Could you check a few things on this model? Use its own coordinates, in mm. A direction names the side the tool comes from. Round coordinates to 2 decimals unless told otherwise and drop trailing zeros. Write each loop counter-clockwise with the first axis right and the second up, starting at its lowest first coordinate (ties: lowest second). Pieces come first, ordered by that corner, then holes. Notation, with made-up numbers: (84, 58) - (123, 58) arc R19 ccw to (123, 79) - close; hole circle Ø4 at (39.25, 5.25). An arc over 180 degrees is marked (long way). Put each result on its own line as item: value.
from build123d import *

# Parameters (mm, degrees)
BOX023_W                 = 4
BOX023_H                 = 9
BOX023_DEPTH             = 3
PRISM015_DEPTH           = 10
PRISM015_ROLL_ANGLE      = -90.000052
PRISM015_PITCH_ANGLE     = -59.999967
PRISM015_PLACEMENT_ANGLE = 90.000052
CYLINDER032_R            = 1.75
CYLINDER032_DEPTH        = 68
CYLINDER032_PITCH_ANGLE  = 90
BOX022_W                 = 6
BOX022_H                 = 9
BOX022_DEPTH             = 11
CHAMFER020_SIZE          = 1.5
FILLET015_R              = 1.5
BOX021_W                 = 12
BOX021_H                 = 16
BOX021_DEPTH             = 10
CYLINDER033_R            = 2
CYLINDER033_DEPTH        = 15
PAD035009_DEPTH          = 35
CYLINDER034_R            = 1.75
CYLINDER034_DEPTH        = 50
PRISM012_DEPTH           = 10
SKETCH031_W              = 88
SKETCH031_H              = 83
PAD035007_DEPTH          = 2
SKETCH032_W              = 58
SKETCH032_H              = 72
PAD035008_DEPTH          = 6
BOX020_W                 = 92
BOX020_H                 = 87
BOX020_DEPTH             = 6
CHAMFER019_SIZE          = 1


with BuildPart() as cubo022:
    # Box023 → Box023 (new body)
    with BuildSketch(Plane(origin=(-29.75, -4.5, 23), x_dir=(1, 0, 0), z_dir=(0, 0, 1))):
        with Locations((2, 4.5)):
            Rectangle(BOX023_W, BOX023_H)
    extrude(amount=BOX023_DEPTH)


with BuildPart() as prisma015:
    # Prism015 → Prism015 (new body)
    with BuildSketch(Plane.XY):
        Polygon((3.25, 0), (1.625, 2.814583), (-1.625, 2.814583), (-3.25, 0), (-1.625, -2.814583), (1.625, -2.814583), align=None)
    extrude(amount=PRISM015_DEPTH)


with BuildPart() as prisma015_1:
    # Prism015 roll: moved
    add(prisma015.part.rotate(Axis((0, 0, 0), (1, 0, 0)), PRISM015_ROLL_ANGLE))


with BuildPart() as prisma015_2:
    # Prism015 pitch: moved
    add(prisma015_1.part.rotate(Axis((0, 0, 0), (0, 1, 0)), PRISM015_PITCH_ANGLE))


with BuildPart() as prisma015_3:
    # Prism015 placement: moved
    add(prisma015_2.part.moved(Location((-17.5, 0, 18))).rotate(Axis((-17.5, 0, 18), (0, 0, 1)), PRISM015_PLACEMENT_ANGLE))


with BuildPart() as cilindro027:
    # Cylinder032 → Cylinder032 (new body)
    with BuildSketch(Plane.XY):
        Circle(CYLINDER032_R)
    extrude(amount=CYLINDER032_DEPTH)


with BuildPart() as cilindro027_1:
    # Cylinder032 pitch: moved
    add(cilindro027.part.rotate(Axis((0, 0, 0), (0, 1, 0)), CYLINDER032_PITCH_ANGLE))


with BuildPart() as cilindro027_2:
    # Cylinder032 placement: moved
    add(cilindro027_1.part.moved(Location((-34, 0, 18))))


with BuildPart() as fusion039:
    # Box022 → Box022 (new body)
    with BuildSketch(Plane(origin=(-28.75, -4.5, 14), x_dir=(1, 0, 0), z_dir=(0, 0, 1))):
        with Locations((3, 4.5)):
            Rectangle(BOX022_W, BOX022_H)
    extrude(amount=BOX022_DEPTH)

    # Cut050: cut Cilindro027
    add(cilindro027_2.part, mode=Mode.SUBTRACT)

    # Chamfer020
    chamfer020_edges = [fusion039.edges().sort_by_distance(p)[0] for p in [
        (-28.75, 0, 14),
    ]]
    chamfer(chamfer020_edges, length=CHAMFER020_SIZE)

    # Fillet015
    fillet015_edges = [fusion039.edges().sort_by_distance(p)[0] for p in [
        (-25, -4.5, 14),
        (-25, 4.5, 14),
    ]]
    fillet(fillet015_edges, radius=FILLET015_R)

    # Cut051: cut Prisma015
    add(prisma015_3.part, mode=Mode.SUBTRACT)

    # Fusion039: union Cubo022
    add(cubo022.part)


with BuildPart() as fusion039_1:
    # Fusion039 placement: moved
    add(fusion039.part.moved(Location((-15, -0.5, -1))))


with BuildPart() as fusion044:
    # Part__Mirroring048: instance of Fusion039
    add(fusion039_1.part.mirror(Plane(origin=(0, 0, 0), x_dir=(0, -1, 0), z_dir=(1, 0, 0))))

    # Fusion044: union Fusion039
    add(fusion039_1.part)


with BuildPart() as fusion044_1:
    # Fusion044 placement: moved
    add(fusion044.part.moved(Location((0, 0, 1.5))))


with BuildPart() as back_cover_hole:
    # Box021 → Box021 (new body)
    with BuildSketch(Plane(origin=(-6, 30, 22), x_dir=(1, 0, 0), z_dir=(0, 0, 1))):
        with Locations((6, 8)):
            Rectangle(BOX021_W, BOX021_H)
    extrude(amount=BOX021_DEPTH)


with BuildPart() as fusion043:
    # Cylinder033 → Cylinder033 (new body)
    with BuildSketch(Plane(origin=(-7, 26, 17), x_dir=(1, 0, 0), z_dir=(0, 0, 1))):
        Circle(CYLINDER033_R)
    extrude(amount=CYLINDER033_DEPTH)

    # Fusion043: union back_cover_hole
    add(back_cover_hole.part)


with BuildPart() as hole_cover:
    # Sketch033 → Pad035009 (new body)
    with BuildSketch(Plane.XY.offset(40)):
        with BuildLine():
            Line((-7, 7), (7, 7))
            ThreePointArc((8.5, 5.5), (8.06066, 6.56066), (7, 7))
            Line((8.5, 5.5), (8.5, -16.5))
            ThreePointArc((7, -18), (8.06066, -17.56066), (8.5, -16.5))
            Line((7, -18), (-7, -18))
            ThreePointArc((-8.5, -16.5), (-8.06066, -17.56066), (-7, -18))
            Line((-8.5, -16.5), (-8.5, 5.5))
            ThreePointArc((-7, 7), (-8.06066, 6.56066), (-8.5, 5.5))
        make_face()
    extrude(amount=-PAD035009_DEPTH)


with BuildPart() as cilindro:
    # Cylinder034 → Cylinder034 (new body)
    with BuildSketch(Plane.XY.offset(-15)):
        Circle(CYLINDER034_R)
    extrude(amount=CYLINDER034_DEPTH)


with BuildPart() as screw_nut_hole:
    # Prism012 → Prism012 (new body)
    with BuildSketch(Plane.XY):
        Polygon((3.1, 0), (1.55, 2.684679), (-1.55, 2.684679), (-3.1, 0), (-1.55, -2.684679), (1.55, -2.684679), align=None)
    extrude(amount=PRISM012_DEPTH)

    # Fusion041: union Cilindro
    add(cilindro.part)


with BuildPart() as screw_nut_hole_1:
    # Fusion041 placement: moved
    add(screw_nut_hole.part.moved(Location((37, 29.565, 9.5))))


with BuildPart() as part_mirroring049:
    # Part__Mirroring049: instance of screw_nut_hole
    add(screw_nut_hole_1.part.mirror(Plane(origin=(0, 0, 0), x_dir=(0, -1, 0), z_dir=(1, 0, 0))))


with BuildPart() as part_mirroring050:
    # Part__Mirroring050: instance of Part__Mirroring049
    add(part_mirroring049.part.mirror(Plane(origin=(0, 0, 0), x_dir=(1, 0, 0), z_dir=(0, 1, 0))))


with BuildPart() as screw_nuts_holes:
    # Part__Mirroring051: instance of screw_nut_hole
    add(screw_nut_hole_1.part.mirror(Plane(origin=(0, 0, 0), x_dir=(1, 0, 0), z_dir=(0, 1, 0))))

    # Fusion042: union screw_nut_hole, Part__Mirroring049, Part__Mirroring050
    add(screw_nut_hole_1.part)
    add(part_mirroring049.part)
    add(part_mirroring050.part)


with BuildPart() as screw_nuts_holes_1:
    # Fusion042 placement: moved
    add(screw_nuts_holes.part.moved(Location((0, 0, 7.5))))


with BuildPart() as pad035007:
    # Sketch031 → Pad035007 (new body)
    with BuildSketch(Plane(origin=(0, 0, 23), x_dir=(1, 0, 0), z_dir=(0, 0, -1))):
        Rectangle(SKETCH031_W, SKETCH031_H)
    extrude(amount=-PAD035007_DEPTH)


with BuildPart() as down_cover_base:
    # Sketch032 → Pad035008 (new body)
    with BuildSketch(Plane(origin=(0, 0, 23), x_dir=(1, 0, 0), z_dir=(0, 0, -1))):
        Rectangle(SKETCH032_W, SKETCH032_H)
    extrude(amount=-PAD035008_DEPTH)

    # Fusion037: union Pad035007
    add(pad035007.part)


with BuildPart() as down_cover_base_1:
    # Fusion037 placement: moved
    add(down_cover_base.part.moved(Location((0, 0, -1))))


with BuildPart() as cover:
    # Box020 → Box020 (new body)
    with BuildSketch(Plane(origin=(-46, -43, 23), x_dir=(1, 0, 0), z_dir=(0, 0, 1))):
        with Locations((46, 43.5)):
            Rectangle(BOX020_W, BOX020_H)
    extrude(amount=BOX020_DEPTH)

    # Chamfer019
    chamfer019_edges = [cover.edges().sort_by_distance(p)[0] for p in [
        (-46, -43, 26),
        (-46, 0.5, 29),
        (-46, 44, 26),
        (46, -43, 26),
        (46, 0.5, 29),
        (46, 44, 26),
        (0, -43, 29),
        (0, 44, 29),
    ]]
    chamfer(chamfer019_edges, length=CHAMFER019_SIZE)

    # Cut052: cut down_cover_base
    add(down_cover_base_1.part, mode=Mode.SUBTRACT)

    # Cut053: cut screw_nuts_holes
    add(screw_nuts_holes_1.part, mode=Mode.SUBTRACT)

    # Cut054: cut hole_cover
    add(hole_cover.part, mode=Mode.SUBTRACT)

    # Cut055: cut Fusion043
    add(fusion043.part, mode=Mode.SUBTRACT)


with BuildPart() as cover_1:
    # Cut055 placement: moved
    add(cover.part.moved(Location((0, -0.5, 0))))

    # Fusion045: union Fusion044
    add(fusion044_1.part)


with BuildPart() as cover_2:
    # Fusion045 placement: moved
    add(cover_1.part.moved(Location((0, 0, -1.5))))


solid = cover_2.part
(1) Please list where these lines run through material, in increasing order: probe 1 along Y at (x, z) = (37, 25.9) (3 decimals); probe 2 along X at (y, z) = (17.5, 23.5); probe 3 along Y at (x, z) = (37, 26.8) (3 decimals). Write a range as from..to.
Values found:
probe 1: y = -43.5..-31.815, -28.315..27.315, 30.815..43.5
probe 2: x = -46..-29, 29..46
probe 3: y = -43.2..-31.815, -28.315..27.315, 30.815..43.2
(2) If we mould it in two halves opening along X, with no side actions, what happens to faces 4 (the face through (-37.75, -3, 20)), 5 (the face through (-1, 10, 27.5))? For each: pulls with the +X half, pulls with the -X half, needs draft (parallel to the pull), parting line crosses it, or undercut.
Values found:
face 4: undercut
face 5: needs draft
(3) For faces 1 (the face through (0, 7, 26.5)), 2 (the face through (40.092, -2.926, 15.573)), 3 (the face through (-38.67, 29.59, 26.49)), which set-ups out of +Z, -Z, +X, -X, +Y, -Y let a thin tool reach every point of the face, with its end or its side?
Values found:
face 1: -Z
face 2: none
face 3: +Z, -Z
(4) Imagine slicing it at A-A, the plane x = -24.5. List the corners of the cut face in (y, z) for me.
Values found:
outline: (-43.5, 21.5) - (-42, 21.5) - (-42, 22.5) - (-36.5, 22.5) - (-36.5, 26.5) - (35.5, 26.5) - (35.5, 22.5) - (41, 22.5) - (41, 21.5) - (43.5, 21.5) - (43.5, 26.5) - (42.5, 27.5) - (-42.5, 27.5) - (-43.5, 26.5) - close
(5) I'm going to push flat-ended pins straight in: pin 1 (2 mm diameter, centred on y = -5, z = 15, fed in from -X); pin 2 (1.9 mm diameter, centred on x = -41, z = 17.5, fed in from +Y); pin 3 (3 mm diameter, centred on y = -0.5, z = 16, fed in from +X). Where does each tip first touch, or does it pass through?
Values found:
pin 1: stops at x = -43.75
pin 2: stops at y = 4
pin 3: stops at x = 43.75
(6) Imagine slicing it at C-C, the plane y = -23.5. List the corners of the cut face in (x, z) for me, then the cut area to 3 significant figures.
Values found:
outline: (-46, 21.5) - (-44, 21.5) - (-44, 22.5) - (-29, 22.5) - (-29, 26.5) - (29, 26.5) - (29, 22.5) - (44, 22.5) - (44, 21.5) - (46, 21.5) - (46, 26.5) - (45, 27.5) - (-45, 27.5) - (-46, 26.5) - close
area: 231 mm^2
(7) Imagine slicing it at B-B, the plane y = -0.5. Give the number of separate pieces and of enclosed holes in the cut face, then the cut area to 3 significant figures.
Values found:
separate pieces: 4
enclosed holes: 0
area: 264 mm^2
